```python
from build123d import *

# Parameters (mm, degrees)
SKETCH1_W               = 8
SKETCH1_H               = 8
BOSS_EXTRUDE1_DEPTH     = 1
FILLET1_R               = 2
BOSS_EXTRUDE2_DEPTH     = 1.25
CUT_EXTRUDE1_DEPTH      = 13.369316877
CUT_EXTRUDE1_DEPTH_BACK = 13.369316877
SKETCH3_R               = 1.5


with BuildPart() as part:
    # Sketch1 → Boss-Extrude1 (new, symmetric)
    with BuildSketch(Plane.XY):
        Rectangle(SKETCH1_W, SKETCH1_H)
    extrude(amount=BOSS_EXTRUDE1_DEPTH, both=True)

    # Fillet1
    fillet1_edges = [part.edges().sort_by_distance(p)[0] for p in [
        (-4, 4, 0),
        (4, 4, 0),
        (4, -4, 0),
        (-4, -4, 0),
    ]]
    fillet(fillet1_edges, radius=FILLET1_R)

    # Sketch2 → Boss-Extrude2 (add, symmetric)
    with BuildSketch(Plane(origin=(0, 0, 0), x_dir=(0, 0, -1), z_dir=(1, 0, 0))):
        with BuildLine():
            Line((1, 3), (8, 3))
            ThreePointArc((8, 3), (11, 0), (8, -3))
            Line((8, -3), (1, -3))
            Line((1, -3), (1, 3))
        make_face()
    extrude(amount=BOSS_EXTRUDE2_DEPTH, both=True)

    # Sketch3 → Cut-Extrude1 (cut, two sides: drawn at the far end of the back side and taken through both)
    with BuildSketch(Plane(origin=(0, 0, 0), x_dir=(0, 0, -1), z_dir=(1, 0, 0)).offset(-CUT_EXTRUDE1_DEPTH_BACK)):
        with Locations((8, 0)):
            Circle(SKETCH3_R)
    extrude(amount=CUT_EXTRUDE1_DEPTH + CUT_EXTRUDE1_DEPTH_BACK, mode=Mode.SUBTRACT)


solid = part.part
```
Design review of the part built by this model. Coordinates are the model's own, in mm. A direction names the side the tool comes from. Coordinates: 2 decimals unless noted, no trailing zeros. Order: outer loops, then holes, each group sorted by start corner. A loop starts at its lowest first (then second) coordinate and runs counter-clockwise, first axis right, second up.
1) Clearance check with flat-ended pins moving along their axes: pin 1 (2 mm diameter, centred on x = 0.5, z = -6, fed in from +Y); pin 2 (3 mm diameter, centred on x = -0.5, z = -5.5, fed in from -Y); pin 3 (1 mm diameter, centred on y = 1.5, z = -7.5, fed in from +X). State where each tip first meets the part, or that it passes through.
2) Take a section at B-B, the plane z = -7.75. Give the boundary of the cut face in (x, y).
3) Take a section at A-A, the plane y = 0. Give the boundary of the cut face in (x, z), and give its area (3 significant figures).
4) Take a section at C-C, the plane y = 2.75. Give the boundary of the cut face in (x, z).
5) Mouldability with a two-part tool opening along Y and no side actions: class faces 1 (the flat face through (-4, 0, 0)), 2 (the cylindrical face through (-0.02, 0.07, -6.5)), 3 (the flat face through (0, 4, 0)) as +Y half, -Y half, draft (parallel to the pull), parting line (faces both ways), or undercut.
6) Take a section at D-D, the plane y = -1. Give the boundary of the cut face in (x, z), and give its area (3 significant figures).
7) For faces 4 (the flat face through (-1.25, 0, -5)), 5 (the flat face through (0, 3, -4)), 6 (the cylindrical face through (3.43, -3.4, 0.01)), 7 (the flat face through (0, -3, -5)), 8 (the flat face through (1.25, 0, -5)), list the 3-axis set-ups (+Z, -Z, +X, -X, +Y, -Y) from which the entire face can be reached by the end or side of a thin tool; tool diameter is ignored.
8) Wall thickness on line 1 along Y through (x, z) = (-0.25, -8); line 2 along Y through (x, z) = (-0.75, -5.5); line 3 along Z through (x, y) = (-2.5, 3.25): over which ranges is each line inside the solid? List them lowest first.
Returned:
1. pin 1: stops at y = 3
1. pin 2: stops at y = -3
1. pin 3: stops at x = 1.25
2. outline: (-1.25, -3) - (1.25, -3) - (1.25, -1.48) - (-1.25, -1.48) - close; (-1.25, 1.48) - (1.25, 1.48) - (1.25, 3) - (-1.25, 3) - close
3. outline: (-4, -1) - (-1.25, -1) - (-1.25, -6.5) - (1.25, -6.5) - (1.25, -1) - (4, -1) - (4, 1) - (-4, 1) - close; (-1.25, -11) - (1.25, -11) - (1.25, -9.5) - (-1.25, -9.5) - close
3. area: 33.5 mm2
4. outline: (-3.85, -1) - (-1.25, -1) - (-1.25, -9.2) - (1.25, -9.2) - (1.25, -1) - (3.85, -1) - (3.85, 1) - (-3.85, 1) - close
5. face 1: draft
5. face 2: undercut
5. face 3: +Y half
6. outline: (-4, -1) - (-1.25, -1) - (-1.25, -6.88) - (1.25, -6.88) - (1.25, -1) - (4, -1) - (4, 1) - (-4, 1) - close; (-1.25, -10.83) - (1.25, -10.83) - (1.25, -9.12) - (-1.25, -9.12) - close
6. area: 35.0 mm2
7. face 4: -Z, -X, +Y, -Y
7. face 5: -Z, +X, -X, +Y
7. face 6: +Z, -Z, +X, -Y
7. face 7: -Z, +X, -X, -Y
7. face 8: -Z, +X, +Y, -Y
8. line 1: y = -3 to -1.5, 1.5 to 3
8. line 2: y = -3 to 3
8. line 3: z = -1 to 1
